```python
from build123d import *

# Parameters (mm, degrees)
F1_DEPTH = 762


with BuildPart() as f1:
    # F0 (on Front) → F1 (new body, symmetric)
    with BuildSketch(Plane.XZ):
        with BuildLine():
            Line((-38.1, -50.8), (38.1, -50.8))
            ThreePointArc((38.1, -50.8), (47.080256, -47.080256), (50.8, -38.1))
            Line((50.8, -38.1), (50.8, 38.1))
            ThreePointArc((50.8, 38.1), (47.080256, 47.080256), (38.1, 50.8))
            Line((38.1, 50.8), (-38.1, 50.8))
            ThreePointArc((-38.1, 50.8), (-47.080256, 47.080256), (-50.8, 38.1))
            Line((-50.8, 38.1), (-50.8, -38.1))
            ThreePointArc((-50.8, -38.1), (-47.080256, -47.080256), (-38.1, -50.8))
        make_face()
        with BuildLine():
            ThreePointArc((44.45, -38.1), (42.590128, -42.590128), (38.1, -44.45))
            Line((38.1, -44.45), (-38.1, -44.45))
            ThreePointArc((-38.1, -44.45), (-42.590128, -42.590128), (-44.45, -38.1))
            Line((-44.45, -38.1), (-44.45, 38.1))
            ThreePointArc((-44.45, 38.1), (-42.590128, 42.590128), (-38.1, 44.45))
            Line((-38.1, 44.45), (38.1, 44.45))
            ThreePointArc((38.1, 44.45), (42.590128, 42.590128), (44.45, 38.1))
            Line((44.45, 38.1), (44.45, -38.1))
        make_face(mode=Mode.SUBTRACT)
    extrude(amount=F1_DEPTH, both=True)


solid = f1.part
```
Input: part model. Units: mm. Frame: model coordinates. A direction names the side the tool comes from. Coordinates: 2 decimals unless noted, no trailing zeros. Loops run counter-clockwise (first coordinate to the right, second up) from the corner with the lowest first, then second, coordinate; pieces in that order, holes last.
Q1. Mould query, pull axis Z, two halves, no side actions, for faces 3 (the flat face through (50.8, -11, -1)), 4 (the flat face through (1, -11, 50.8)), 5 (the flat face through (-1, -11, 44.45)). Classes: +Z half, -Z half, draft (parallel to the pull), parting line (faces both ways), or undercut.
Results are:
face 3: draft
face 4: +Z half
face 5: undercut
Q2. Set-up query: faces 1 (the flat face through (-1, -11, -50.8)), 2 (the flat face through (-44.45, -11, -1)). Return all of +Z, -Z, +X, -X, +Y, -Y with unobstructed straight access to the full face (end or side cutting, diameter ignored); none if empty.
Results are:
face 1: -Z, +X, -X, +Y, -Y
face 2: +Y, -Y
Q3. Line query: line 1 along Z through (x, y) = (20, -1); line 2 along X through (y, z) = (550, 41.5). Output: solid intervals per line, ascending.
Results are:
line 1: z = -50.8 to -44.45, 44.45 to 50.8
line 2: x = -50.34 to -43.46, 43.46 to 50.34
Q4. Section B-B, the plane y = 68. Return the cut outline in (x, z).
Results are:
outline: (-50.8, -38.1) arc R12.7 ccw to (-38.1, -50.8) - (38.1, -50.8) arc R12.7 ccw to (50.8, -38.1) - (50.8, 38.1) arc R12.7 ccw to (38.1, 50.8) - (-38.1, 50.8) arc R12.7 ccw to (-50.8, 38.1) - close; hole (-44.45, -38.1) arc R6.35 ccw to (-38.1, -44.45) - (38.1, -44.45) arc R6.35 ccw to (44.45, -38.1) - (44.45, 38.1) arc R6.35 ccw to (38.1, 44.45) - (-38.1, 44.45) arc R6.35 ccw to (-44.45, 38.1) - close
Q5. Section A-A, the plane z = 22.5. Return the cut outline in (x, y).
Results are:
outline: (-50.8, -762) - (-44.45, -762) - (-44.45, 762) - (-50.8, 762) - close; (44.45, -762) - (50.8, -762) - (50.8, 762) - (44.45, 762) - close
Q6. Section C-C, the plane x = 6.5. Return the cut outline in (y, z).
Results are:
outline: (-762, -50.8) - (762, -50.8) - (762, -44.45) - (-762, -44.45) - close; (-762, 44.45) - (762, 44.45) - (762, 50.8) - (-762, 50.8) - close
